```python
from build123d import *

# Parameters (mm, degrees)
SZKIC1_W                    = 300
SZKIC1_H                    = 140
DODANIE_WYCI_GNI_CIE1_DEPTH = 15
DODANIE_WYCI_GNI_CIE1_DRAFT = -45
SZKIC2_W                    = 300
SZKIC2_H                    = 70
WYTNIJ_WYCI_GNI_CIE1_DEPTH  = 15
SZKIC3_W                    = 10
SZKIC3_H                    = 12
WYTNIJ_WYCI_GNI_CIE2_DEPTH  = 108
ZAOKR_GLENIE1_R             = 10


with BuildPart() as part:
    # Szkic1 → Dodanie-wyciągnięcie1 (with draft: the straight prism first)
    with BuildSketch(Plane.XY):
        Rectangle(SZKIC1_W, SZKIC1_H)
    extrude(amount=DODANIE_WYCI_GNI_CIE1_DEPTH)
    # Dodanie-wyciągnięcie1: the draft: its side faces are tilted about the plane it starts from
    dodanie_wyci_gni_cie1_sides = [part.faces().sort_by_distance(p)[0] for p in [
        (0, -70, 7.5),
        (150, 0, 7.5),
        (0, 70, 7.5),
        (-150, 0, 7.5),
    ]]
    draft(dodanie_wyci_gni_cie1_sides, Plane.XY, DODANIE_WYCI_GNI_CIE1_DRAFT)

    # Szkic2 → Wytnij-wyciągnięcie1 (cut)
    with BuildSketch(Plane(origin=(0, 0, 2), x_dir=(-1, 0, 0), z_dir=(0, 0, -1))):
        with Locations((0, 35)):
            Rectangle(SZKIC2_W, SZKIC2_H)
    extrude(amount=-WYTNIJ_WYCI_GNI_CIE1_DEPTH, mode=Mode.SUBTRACT)

    # Szkic3 → Wytnij-wyciągnięcie2 (cut)
    with BuildSketch(Plane(origin=(0, 0, 0), x_dir=(1, 0, 0), z_dir=(0, 1, 0))):
        with Locations((-140, -8)):
            Rectangle(SZKIC3_W, SZKIC3_H)
        with Locations((-127.8, -8)):
            Rectangle(SZKIC3_W, SZKIC3_H)
        with Locations((-115.6, -8)):
            Rectangle(SZKIC3_W, SZKIC3_H)
        with Locations((-103.4, -8)):
            Rectangle(SZKIC3_W, SZKIC3_H)
        with Locations((-91.2, -8)):
            Rectangle(SZKIC3_W, SZKIC3_H)
        with Locations((-79, -8)):
            Rectangle(SZKIC3_W, SZKIC3_H)
        with Locations((-66.8, -8)):
            Rectangle(SZKIC3_W, SZKIC3_H)
        with Locations((-54.6, -8)):
            Rectangle(SZKIC3_W, SZKIC3_H)
        with Locations((-42.4, -8)):
            Rectangle(SZKIC3_W, SZKIC3_H)
        with Locations((-30.2, -8)):
            Rectangle(SZKIC3_W, SZKIC3_H)
        with Locations((-18, -8)):
            Rectangle(SZKIC3_W, SZKIC3_H)
        with Locations((-5.8, -8)):
            Rectangle(SZKIC3_W, SZKIC3_H)
        with Locations((6.4, -8)):
            Rectangle(SZKIC3_W, SZKIC3_H)
        with Locations((18.6, -8)):
            Rectangle(SZKIC3_W, SZKIC3_H)
        with Locations((30.8, -8)):
            Rectangle(SZKIC3_W, SZKIC3_H)
        with Locations((43, -8)):
            Rectangle(SZKIC3_W, SZKIC3_H)
        with Locations((55.2, -8)):
            Rectangle(SZKIC3_W, SZKIC3_H)
        with Locations((67.4, -8)):
            Rectangle(SZKIC3_W, SZKIC3_H)
        with Locations((79.6, -8)):
            Rectangle(SZKIC3_W, SZKIC3_H)
        with Locations((91.8, -8)):
            Rectangle(SZKIC3_W, SZKIC3_H)
        with Locations((104, -8)):
            Rectangle(SZKIC3_W, SZKIC3_H)
        with Locations((116.2, -8)):
            Rectangle(SZKIC3_W, SZKIC3_H)
        with Locations((128.4, -8)):
            Rectangle(SZKIC3_W, SZKIC3_H)
        with Locations((140.6, -8)):
            Rectangle(SZKIC3_W, SZKIC3_H)
    extrude(amount=-WYTNIJ_WYCI_GNI_CIE2_DEPTH, mode=Mode.SUBTRACT)

    # Zaokrąglenie1
    # the kernel refuses this fillet: 10 mm, written as the material it takes off along each edge
    with BuildSketch(Plane(origin=(-145.857864376, 65.857864376, 10), x_dir=(-0.35740674433659364, 0.8628562094610169, 0.3574067443365923), z_dir=(-0.2705980500730978, 0.2705980500730978, -0.9238795325112871))) as zaokr_glenie1_piece_1_section:
        Polygon((-13.907299812, -13.907299812), (13.907299812, -13.907299812), (13.907299812, 13.907299812), (-13.907299812, 13.907299812), align=None)
    zaokr_glenie1_piece_1 = extrude(amount=13.907299812, mode=Mode.PRIVATE)
    zaokr_glenie1_piece_1 = split(zaokr_glenie1_piece_1, bisect_by=Plane(origin=(-145.857864376, 65.857864376, 10), z_dir=(0, 1, 0)), keep=Keep.TOP, mode=Mode.PRIVATE)
    zaokr_glenie1_piece_1 = split(zaokr_glenie1_piece_1, bisect_by=Plane(origin=(-145.857864376, 65.857864376, 10), z_dir=(-1, 0, 0)), keep=Keep.TOP, mode=Mode.PRIVATE)
    zaokr_glenie1_piece_1 = split(zaokr_glenie1_piece_1, bisect_by=Plane(origin=(-145.857864376, 65.857864376, 10), z_dir=(0.5773502691896265, -0.5773502691896265, -0.5773502691896244)), keep=Keep.TOP, mode=Mode.PRIVATE)
    zaokr_glenie1_piece_1 = split(zaokr_glenie1_piece_1, bisect_by=Plane(origin=(-152.928932188, 65.857864376, 2.928932188), z_dir=(0.7071067811865462, 0, 0.7071067811865488)), keep=Keep.TOP, mode=Mode.PRIVATE)
    zaokr_glenie1_piece_1 = split(zaokr_glenie1_piece_1, bisect_by=Plane(origin=(-145.857864376, 65.857864376, 0), z_dir=(0, 0, 1)), keep=Keep.TOP, mode=Mode.PRIVATE)
    zaokr_glenie1_piece_1 = split(zaokr_glenie1_piece_1, bisect_by=Plane(origin=(-145.857864376, 72.928932188, 2.928932188), z_dir=(0, -0.7071067811865462, 0.7071067811865488)), keep=Keep.TOP, mode=Mode.PRIVATE)
    zaokr_glenie1_piece_1 = zaokr_glenie1_piece_1 - Plane(origin=(-145.857864376, 65.857864376, 10), x_dir=(0.2705980500730978, -0.2705980500730978, 0.9238795325112871), z_dir=(-0.35740674433659364, 0.8628562094610169, 0.3574067443365923)) * Sphere(ZAOKR_GLENIE1_R, mode=Mode.PRIVATE)
    add(zaokr_glenie1_piece_1, mode=Mode.SUBTRACT)
    with BuildSketch(Plane(origin=(145.857864376, 65.857864376, 10), x_dir=(-0.7071067811865475, 0.7071067811865475, 0), z_dir=(0.2705980500730978, 0.2705980500730978, -0.9238795325112871))) as zaokr_glenie1_piece_2_section:
        Polygon((-13.907299812, -13.907299812), (13.907299812, -13.907299812), (13.907299812, 13.907299812), (-13.907299812, 13.907299812), align=None)
    zaokr_glenie1_piece_2 = extrude(amount=13.907299812, mode=Mode.PRIVATE)
    zaokr_glenie1_piece_2 = split(zaokr_glenie1_piece_2, bisect_by=Plane(origin=(145.857864376, 65.857864376, 10), z_dir=(0, 1, 0)), keep=Keep.TOP, mode=Mode.PRIVATE)
    zaokr_glenie1_piece_2 = split(zaokr_glenie1_piece_2, bisect_by=Plane(origin=(145.857864376, 65.857864376, 10), z_dir=(-0.5773502691896265, -0.5773502691896265, -0.5773502691896244)), keep=Keep.TOP, mode=Mode.PRIVATE)
    zaokr_glenie1_piece_2 = split(zaokr_glenie1_piece_2, bisect_by=Plane(origin=(145.857864376, 65.857864376, 10), z_dir=(1, 0, 0)), keep=Keep.TOP, mode=Mode.PRIVATE)
    zaokr_glenie1_piece_2 = split(zaokr_glenie1_piece_2, bisect_by=Plane(origin=(145.857864376, 65.857864376, 0), z_dir=(0, 0, 1)), keep=Keep.TOP, mode=Mode.PRIVATE)
    zaokr_glenie1_piece_2 = split(zaokr_glenie1_piece_2, bisect_by=Plane(origin=(152.928932188, 65.857864376, 2.928932188), z_dir=(-0.7071067811865462, 0, 0.7071067811865488)), keep=Keep.TOP, mode=Mode.PRIVATE)
    zaokr_glenie1_piece_2 = split(zaokr_glenie1_piece_2, bisect_by=Plane(origin=(145.857864376, 72.928932188, 2.928932188), z_dir=(0, -0.7071067811865462, 0.7071067811865488)), keep=Keep.TOP, mode=Mode.PRIVATE)
    zaokr_glenie1_piece_2 = zaokr_glenie1_piece_2 - Plane(origin=(145.857864376, 65.857864376, 10), x_dir=(-0.2705980500730978, -0.2705980500730978, 0.9238795325112871), z_dir=(-0.7071067811865475, 0.7071067811865475, 0)) * Sphere(ZAOKR_GLENIE1_R, mode=Mode.PRIVATE)
    add(zaokr_glenie1_piece_2, mode=Mode.SUBTRACT)
    with BuildSketch(Plane(origin=(-150, 65.857864376, 0), x_dir=(-0.7071067811865438, 0, 0.7071067811865511), z_dir=(0, -1, 0))) as zaokr_glenie1_piece_3:
        with BuildLine():
            CenterArc((ZAOKR_GLENIE1_R * 0.414213562373, -ZAOKR_GLENIE1_R), ZAOKR_GLENIE1_R, 90, 45)
            Line((-ZAOKR_GLENIE1_R * 0.292893218813, -ZAOKR_GLENIE1_R * 0.292893218813), (0, 0))
            Line((0, 0), (ZAOKR_GLENIE1_R * 0.414213562373, 0))
        make_face()
    extrude(amount=146.213203436, mode=Mode.SUBTRACT)
    with BuildSketch(Plane(origin=(145.857864376, 70, 0), x_dir=(0, -1, 0), z_dir=(-1, 0, 0))) as zaokr_glenie1_piece_4:
        with BuildLine():
            CenterArc((ZAOKR_GLENIE1_R * 0.414213562373, ZAOKR_GLENIE1_R), ZAOKR_GLENIE1_R, 225, 45)
            Line((-ZAOKR_GLENIE1_R * 0.292893218813, ZAOKR_GLENIE1_R * 0.292893218813), (0, 0))
            Line((0, 0), (ZAOKR_GLENIE1_R * 0.414213562373, 0))
        make_face()
    extrude(amount=291.715728753, mode=Mode.SUBTRACT)
    with BuildSketch(Plane(origin=(150, -80.355339059, 0), x_dir=(-1, 0, 0), z_dir=(0, 1, 0))) as zaokr_glenie1_piece_5:
        with BuildLine():
            CenterArc((ZAOKR_GLENIE1_R * 0.414213562373, ZAOKR_GLENIE1_R), ZAOKR_GLENIE1_R, 225, 45)
            Line((-ZAOKR_GLENIE1_R * 0.292893218813, ZAOKR_GLENIE1_R * 0.292893218813), (0, 0))
            Line((0, 0), (ZAOKR_GLENIE1_R * 0.414213562373, 0))
        make_face()
    extrude(amount=146.213203436, mode=Mode.SUBTRACT)
    with BuildSketch(Plane(origin=(141.666666667, -61.666666667, -8.333333333), x_dir=(-0.8164965809277256, -0.40824829046386363, 0.40824829046386335), z_dir=(0.5773502691896265, -0.5773502691896265, 0.5773502691896244))) as zaokr_glenie1_piece_6:
        with BuildLine():
            CenterArc((ZAOKR_GLENIE1_R * 0.57735026919, -ZAOKR_GLENIE1_R), ZAOKR_GLENIE1_R, 90, 60)
            Line((-ZAOKR_GLENIE1_R * 0.288675134595, -ZAOKR_GLENIE1_R * 0.5), (0, 0))
            Line((0, 0), (ZAOKR_GLENIE1_R * 0.57735026919, 0))
        make_face()
    extrude(amount=54.848275573, mode=Mode.SUBTRACT)
    with BuildSketch(Plane(origin=(-141.666666667, -61.666666667, -8.333333333), x_dir=(0.8164965809277256, -0.40824829046386546, 0.40824829046386146), z_dir=(-0.5773502691896265, -0.5773502691896265, 0.5773502691896244))) as zaokr_glenie1_piece_7:
        with BuildLine():
            CenterArc((ZAOKR_GLENIE1_R * 0.57735026919, ZAOKR_GLENIE1_R), ZAOKR_GLENIE1_R, 210, 60)
            Line((-ZAOKR_GLENIE1_R * 0.288675134595, ZAOKR_GLENIE1_R * 0.5), (0, 0))
            Line((0, 0), (ZAOKR_GLENIE1_R * 0.57735026919, 0))
        make_face()
    extrude(amount=54.848275573, mode=Mode.SUBTRACT)
    with BuildSketch(Plane(origin=(-150.571909584, 70.571909584, 0.571909584), x_dir=(-0.4082482904638678, -0.8164965809277256, 0.40824829046385913), z_dir=(-0.5773502691896265, 0.5773502691896265, 0.5773502691896244))) as zaokr_glenie1_piece_8:
        with BuildLine():
            CenterArc((ZAOKR_GLENIE1_R * 0.57735026919, ZAOKR_GLENIE1_R), ZAOKR_GLENIE1_R, 210, 60)
            Line((-ZAOKR_GLENIE1_R * 0.288675134595, ZAOKR_GLENIE1_R * 0.5), (0, 0))
            Line((0, 0), (ZAOKR_GLENIE1_R * 0.57735026919, 0))
        make_face()
    extrude(amount=39.423942386, mode=Mode.SUBTRACT)
    with BuildSketch(Plane(origin=(150.571909584, 70.571909584, 0.571909584), x_dir=(0.4082482904638637, -0.8164965809277256, 0.4082482904638634), z_dir=(0.5773502691896265, 0.5773502691896265, 0.5773502691896244))) as zaokr_glenie1_piece_9:
        with BuildLine():
            CenterArc((ZAOKR_GLENIE1_R * 0.57735026919, -ZAOKR_GLENIE1_R), ZAOKR_GLENIE1_R, 90, 60)
            Line((-ZAOKR_GLENIE1_R * 0.288675134595, -ZAOKR_GLENIE1_R * 0.5), (0, 0))
            Line((0, 0), (ZAOKR_GLENIE1_R * 0.57735026919, 0))
        make_face()
    extrude(amount=39.423942386, mode=Mode.SUBTRACT)


solid = part.part
```
For this review, take the finished solid that the model builds, in its own axes (mm). A direction names the side the tool comes from. Round coordinates to 2 decimals unless told otherwise and drop trailing zeros. Write each loop counter-clockwise with the first axis right and the second up, starting at its lowest first coordinate (ties: lowest second). Pieces come first, ordered by that corner, then holes.
1) Take a section at B-B on y = 40.5. Give the boundary of the cut face in (x, z), then the cut area to 3 significant figures.
Answer below:
outline: (-165, 15) - (-152.93, 2.93) arc R10 ccw to (-145.86, 0) - (145.86, 0) arc R10 ccw to (152.93, 2.93) - (165, 15) - (150, 15) - (150, 2) - (-150, 2) - (-150, 15) - close
area: 821 mm2
2) Take a section at A-A on x = 4.5. Give the boundary of the cut face in (y, z), then the cut area to 3 significant figures.
Answer below:
outline: (-85, 15) - (-84, 14) - (0, 14) - (0, 15) - close; (-72, 2) - (-70, 0) - (65.86, 0) arc R10 ccw to (72.93, 2.93) - (85, 15) - (70, 15) - (70, 2) - close
area: 477 mm2
3) For line 1 along Z through (x, y) = (92.5, -56.5); line 2 along X through (y, z) = (34.5, 14); line 3 along Y through (x, z) = (-146, 10), list the stretches that pass through material, from the lowest coordinate up.
Answer below:
line 1: z = 0 to 2, 14 to 15
line 2: x = -164 to -150, 150 to 164
line 3: y = -80 to 0, 70 to 80
4) Insertion check: pin 1 Ø1.5 at (x, y) = (-119, 2.5) entering from +Z; pin 2 Ø1 at (y, z) = (-5, 5) entering from -X; pin 3 Ø4 at (y, z) = (-31.5, 12) entering from -X. Each pin has a flat end and moves straight along its axis. Give the tip position at first contact, or say it passes through.
Answer below:
pin 1: stops at z = 2
pin 2: stops at x = -155.5
pin 3: stops at x = -164
5) Take a section at C-C on y = -49. State how many separate pieces and enclosed holes the cut face has, then the cut area to 3 significant figures.
Answer below:
separate pieces: 1
enclosed holes: 24
area: 1,840 mm2
6) Mouldability with a two-part tool opening along Z and no side actions: class faces 1 (the face through (-149.735, -0.882, 0.782)), 2 (the face through (-150, 35, 8)), 3 (the face through (-145, -41, 8)) as +Z half, -Z half, draft (parallel to the pull), parting line (faces both ways), or undercut.
Answer below:
face 1: -Z half
face 2: draft
face 3: undercut
7) Machinability: for faces 4 (the face through (-42, -41, 14)), 5 (the face through (156.6, 76.49, 8.44)), which of the approach directions +Z, -Z, +X, -X, +Y, -Y give a long, thin tool a straight path to every point of the face, cutting with its end or side? Answer none if there is none.
Answer below:
face 4: -Y
face 5: -Z, +X, +Y
